The model under review builds one solid part; all positions refer to its coordinate system, in mm. A direction names the side the tool comes from. Coordinates: 2 decimals unless noted, no trailing zeros. Write each loop counter-clockwise with the first axis right and the second up, starting at its lowest first coordinate (ties: lowest second). Pieces come first, ordered by that corner, then holes. Notation, with made-up numbers: M 55,9.5 L 106,9.5 A21 cw 106,46.5 Z; hole C -2,41.25 d8. An arc over 180 degrees is marked long. Answer as CSV lines item,"result". Start each with the question number.
from build123d import *

# Parameters (mm, degrees)
SKETCH1_R           = 15.5
SKETCH1_R_2         = 12.5
EXTRUDE_THIN1_DEPTH = 35
SKETCH2_R           = 15.5
SKETCH2_R_2         = 12.5
EXTRUDE_THIN2_DEPTH = 35
SCALE1_SCALE        = 0.5


with BuildPart() as part:
    # Sketch1 → Extrude-Thin1 (new, symmetric)
    with BuildSketch(Plane.XY):
        Circle(SKETCH1_R)
        Circle(SKETCH1_R_2, mode=Mode.SUBTRACT)
    extrude(amount=EXTRUDE_THIN1_DEPTH, both=True)

    # Sketch2 → Extrude-Thin2 (add, symmetric)
    with BuildSketch(Plane(origin=(0, 0, 0), x_dir=(1, 0, 0), z_dir=(0, 1, 0))):
        Circle(SKETCH2_R)
        Circle(SKETCH2_R_2, mode=Mode.SUBTRACT)
    extrude(amount=EXTRUDE_THIN2_DEPTH, both=True)


with BuildPart() as part_1:
    # Scale1: scaled about (0, 0, 0)
    add(part.part.scale(SCALE1_SCALE))


solid = part_1.part
1) Take a section at B-B on z = -1. Give the boundary of the cut face in (x, y), and give its area (3 significant figures).
2) Mouldability with a two-part tool opening along Y and no side actions: class faces 1 (the cylindrical face through (-5.71, 5.24, -10.57)), 2 (the cylindrical face through (-0.14, -0.09, 6.25)), 3 (the cylindrical face through (5.96, -12.57, -1.88)) as +Y half, -Y half, draft (parallel to the pull), parting line (faces both ways), or undercut.
3) Clearance check with flat-ended pins moving along their axes: pin 1 Ø5 at (x, y) = (4.5, 9.5) entering from -Z; pin 2 Ø10 at (y, z) = (12.5, -7) entering from +X. State where each tip first meets the part, or that it passes through.
4) Take a section at C-C on y = -4. Give the boundary of the cut face in (x, z), and give its area (3 significant figures).
5) Take a section at D-D on z = -5.5. Give the boundary of the cut face in (x, y).
6) Tool access review of faces 4 (the cylindrical face through (5.96, 1.88, -12.57)), 5 (the cylindrical face through (-5.71, -10.57, -5.24)), 6 (the cylindrical face through (3.576, -6.876, 10.817)): name each direction out of +Z, -Z, +X, -X, +Y, -Y from which nothing blocks a thin tool from reaching the whole face with its end or side.
7) To check wall thickness, follow line 1 (Z direction, x = 0, y = -12.75); line 2 (Y direction, x = 3.5, z = -5). State the ranges of each line that lie inside material, in increasing order. Write a range as [from, to].
Results:
1,outline,"M -7.69,-17.5 L -6.17,-17.5 L -6.17,-4.69 A7.75 ccw 6.17,-4.69 L 6.17,-17.5 L 7.69,-17.5 L 7.69,-1 A7.75 ccw 7.69,1 L 7.69,17.5 L 6.17,17.5 L 6.17,4.69 A7.75 ccw -6.17,4.69 L -6.17,17.5 L -7.69,17.5 L -7.69,1 A7.75 ccw -7.69,-1 Z; hole M -6.17,-1 A6.25 ccw 6.17,-1 L 6.17,1 A6.25 ccw -6.17,1 Z"
1,area,"152 mm²"
2,face 1,"parting line"
2,face 2,"undercut"
2,face 3,"draft"
3,pin 1,"stops at z = -7.49"
3,pin 2,"stops at x = 7.49"
4,outline,"M -6.64,-17.5 L -4.8,-17.5 L -4.8,-6.08 A7.75 ccw 4.8,-6.08 L 4.8,-17.5 L 6.64,-17.5 L 6.64,-4 A7.75 ccw 6.64,4 L 6.64,17.5 L 4.8,17.5 L 4.8,6.08 A7.75 ccw -4.8,6.08 L -4.8,17.5 L -6.64,17.5 L -6.64,4 A7.75 ccw -6.64,-4 Z; hole M -4.8,-4 A6.25 ccw 4.8,-4 L 4.8,4 A6.25 ccw -4.8,4 Z"
4,area,"172 mm²"
5,outline,"M -5.46,-17.5 L -2.97,-17.5 L -2.97,-7.16 A7.75 ccw 2.97,-7.16 L 2.97,-17.5 L 5.46,-17.5 L 5.46,-5.5 A7.75 ccw 5.46,5.5 L 5.46,17.5 L 2.97,17.5 L 2.97,7.16 A7.75 ccw -2.97,7.16 L -2.97,17.5 L -5.46,17.5 L -5.46,5.5 A7.75 ccw -5.46,-5.5 Z; hole M -5.46,-3.04 L -5.46,3.04 A6.25 ccw Z; hole M -2.97,-5.5 A6.25 ccw 2.97,-5.5 L 2.97,5.5 A6.25 ccw -2.97,5.5 Z; hole M 5.46,-3.04 A6.25 ccw 5.46,3.04 Z"
6,face 4,"-Z"
6,face 5,"-Y"
6,face 6,"+Z"
7,line 1,"z = [-7.75, -6.25], [6.25, 7.75]"
7,line 2,"y = [-6.91, -5.18], [5.18, 6.91]"
